from build123d import *

# Parameters (mm, degrees)
SKETCH1_W                 = 50.8
SKETCH1_H                 = 50.8
BOSS_EXTRUDE1_DEPTH       = 79.375
CUT_EXTRUDE1_DEPTH        = 3.175
SKETCH3_R                 = 55.5625
CUT_EXTRUDE2_DEPTH        = 108.059192156
F_8_32_TAPPED_HOLE1_D     = 3.4544
F_8_32_TAPPED_HOLE1_DEPTH = 10.70864
F_8_32_TAPPED_HOLE1_TIP   = 1.037806461
F_8_32_TAPPED_HOLE2_D     = 3.4544
F_8_32_TAPPED_HOLE2_DEPTH = 10.70864
F_8_32_TAPPED_HOLE2_TIP   = 1.037806461


with BuildPart() as part:
    # Sketch1 → Boss-Extrude1 (new body)
    with BuildSketch(Plane(origin=(0, 0, 0), x_dir=(1, 0, 0), z_dir=(0, 1, 0))):
        with Locations((25.4, 25.4)):
            Rectangle(SKETCH1_W, SKETCH1_H)
    extrude(amount=BOSS_EXTRUDE1_DEPTH)

    # Sketch2 → Cut-Extrude1 (cut)
    with BuildSketch(Plane(origin=(0, 79.375, 0), x_dir=(1, 0, 0), z_dir=(0, 1, 0))):
        with BuildLine():
            Line((130.016993909, 125.017737196), (134.25782275, 78.573759143))
            ThreePointArc((134.25782275, 78.573759143), (134.034685181, 75.298190088), (132.798116214, 72.256802214))
            ThreePointArc((132.798116214, 72.256802214), (130.01096738, 66.280890285), (128.580118229, 59.844090402))
            ThreePointArc((128.580118229, 59.844090402), (125.846501332, 47.24207899), (120.576283082, 35.473130329))
            ThreePointArc((120.576283082, 35.473130329), (120.013426501, 34.114565768), (119.824473194, 32.656209898))
            ThreePointArc((119.824473194, 32.656209898), (117.90735564, 28.45485307), (113.469501546, 27.177281171))
            ThreePointArc((113.469501546, 27.177281171), (106.116591491, 23.83727612), (106.198458812, 15.761744078))
            ThreePointArc((106.198458812, 15.761744078), (105.465515747, 8.75311664), (98.443142857, 8.166309094))
            ThreePointArc((98.443142857, 8.166309094), (95.25, 9.168506799), (92.056857143, 8.166309094))
            ThreePointArc((92.056857143, 8.166309094), (88.9, 7.1755), (85.743142857, 8.166309094))
            ThreePointArc((85.743142857, 8.166309094), (82.55, 9.168506799), (79.356857143, 8.166309094))
            ThreePointArc((79.356857143, 8.166309094), (76.212257074, 7.175513597), (73.063291467, 8.152345678))
            ThreePointArc((73.063291467, 8.152345678), (69.907489389, 9.140393728), (66.74574768, 8.171520637))
            ThreePointArc((66.74574768, 8.171520637), (63.508942298, 7.175501389), (60.273525168, 8.176020964))
            ThreePointArc((60.273525168, 8.176020964), (57.10532095, 9.149271709), (53.943097961, 8.156759366))
            ThreePointArc((53.943097961, 8.156759366), (50.791625748, 7.175506347), (47.643142857, 8.166309094))
            ThreePointArc((47.643142857, 8.166309094), (44.45, 9.168506799), (41.256857143, 8.166309094))
            ThreePointArc((41.256857143, 8.166309094), (38.1, 7.1755), (34.943142857, 8.166309094))
            ThreePointArc((34.943142857, 8.166309094), (31.75, 9.168506799), (28.556857143, 8.166309094))
            ThreePointArc((28.556857143, 8.166309094), (25.4, 7.1755), (22.243142857, 8.166309094))
            ThreePointArc((22.243142857, 8.166309094), (19.05, 9.168506799), (15.856857143, 8.166309094))
            ThreePointArc((15.856857143, 8.166309094), (8.793588587, 8.793588587), (8.166309094, 15.856857143))
            ThreePointArc((8.166309094, 15.856857143), (9.168506799, 19.05), (8.166309094, 22.243142857))
            ThreePointArc((8.166309094, 22.243142857), (7.1755, 25.4), (8.166309094, 28.556857143))
            ThreePointArc((8.166309094, 28.556857143), (9.168506799, 31.75), (8.166309094, 34.943142857))
            ThreePointArc((8.166309094, 34.943142857), (7.1755, 38.1), (8.166309094, 41.256857143))
            ThreePointArc((8.166309094, 41.256857143), (9.168506799, 44.45), (8.166309094, 47.643142857))
            ThreePointArc((8.166309094, 47.643142857), (7.175506347, 50.791625748), (8.156759366, 53.943097961))
            ThreePointArc((8.156759366, 53.943097961), (9.149271709, 57.10532095), (8.176020964, 60.273525168))
            ThreePointArc((8.176020964, 60.273525168), (7.175501389, 63.508942298), (8.171520637, 66.74574768))
            ThreePointArc((8.171520637, 66.74574768), (9.140393728, 69.907489389), (8.152345678, 73.063291467))
            ThreePointArc((8.152345678, 73.063291467), (7.175513597, 76.212257074), (8.166309094, 79.356857143))
            ThreePointArc((8.166309094, 79.356857143), (9.168506799, 82.55), (8.166309094, 85.743142857))
            ThreePointArc((8.166309094, 85.743142857), (7.1755, 88.9), (8.166309094, 92.056857143))
            ThreePointArc((8.166309094, 92.056857143), (9.168506799, 95.25), (8.166309094, 98.443142857))
            ThreePointArc((8.166309094, 98.443142857), (8.75311664, 105.465515747), (15.761744078, 106.198458812))
            ThreePointArc((15.761744078, 106.198458812), (23.83727612, 106.116591491), (27.177281171, 113.469501546))
            ThreePointArc((27.177281171, 113.469501546), (28.45485307, 117.90735564), (32.656209898, 119.824473194))
            ThreePointArc((32.656209898, 119.824473194), (34.114565768, 120.013426501), (35.473130329, 120.576283082))
            ThreePointArc((35.473130329, 120.576283082), (47.24207899, 125.846501332), (59.844090402, 128.580118229))
            ThreePointArc((59.844090402, 128.580118229), (68.705211612, 130.952457845), (76.452938417, 135.863689229))
            ThreePointArc((76.452938417, 135.863689229), (80.625736152, 138.0725352), (85.345346996, 138.201045691))
            Line((85.345346996, 138.201045691), (125.626948268, 129.926898817))
            ThreePointArc((125.626948268, 129.926898817), (128.63345164, 128.197989094), (130.016993909, 125.017737196))
        make_face()
    extrude(amount=-CUT_EXTRUDE1_DEPTH, mode=Mode.SUBTRACT)

    # Sketch3 → Cut-Extrude2 (cut, through all)
    with BuildSketch(Plane(origin=(0, 79.375, 0), x_dir=(1, 0, 0), z_dir=(0, 1, 0))):
        with Locations((66.675, 66.675)):
            Circle(SKETCH3_R)
    extrude(amount=-CUT_EXTRUDE2_DEPTH, mode=Mode.SUBTRACT)

    # #8-32 Tapped Hole1
    with Locations(Plane(origin=(393.7, -15.875, 0), x_dir=(1, 0, 0), z_dir=(0, 0, 1))):
        with Locations((-300, 82.55), (-240, 82.55), (-180, 82.55), (-60, 82.55), (0, 82.55), (60, 82.55), (120, 82.55), (180, 82.55), (240, 82.55), (-120, 82.55), (-360, 82.55), (300, 82.55), (360, 82.55)):
            Hole(F_8_32_TAPPED_HOLE1_D / 2, depth=F_8_32_TAPPED_HOLE1_DEPTH)
            with Locations((0, 0, -(F_8_32_TAPPED_HOLE1_DEPTH + F_8_32_TAPPED_HOLE1_TIP / 2))):  # 118° drill point
                Cone(0, F_8_32_TAPPED_HOLE1_D / 2, F_8_32_TAPPED_HOLE1_TIP, mode=Mode.SUBTRACT)

    # #8-32 Tapped Hole2
    with Locations(Plane(origin=(0, -15.875, -393.7), x_dir=(0, 0, 1), z_dir=(-1, 0, 0))):
        with Locations((-300, 82.55), (-240, 82.55), (-180, 82.55), (-60, 82.55), (0, 82.55), (60, 82.55), (120, 82.55), (180, 82.55), (240, 82.55), (-120, 82.55), (-360, 82.55), (300, 82.55), (360, 82.55)):
            Hole(F_8_32_TAPPED_HOLE2_D / 2, depth=F_8_32_TAPPED_HOLE2_DEPTH)
            with Locations((0, 0, -(F_8_32_TAPPED_HOLE2_DEPTH + F_8_32_TAPPED_HOLE2_TIP / 2))):  # 118° drill point
                Cone(0, F_8_32_TAPPED_HOLE2_D / 2, F_8_32_TAPPED_HOLE2_TIP, mode=Mode.SUBTRACT)


solid = part.part
Input: part model. Units: mm. Frame: model coordinates. A direction names the side the tool comes from. Coordinates: 2 decimals unless noted, no trailing zeros. Order: outer loops, then holes, each group sorted by start corner. A loop starts at its lowest first (then second) coordinate and runs counter-clockwise, first axis right, second up. Notation, with made-up numbers: M -39.5,57 L -13.5,57 A17 ccw -13.5,88 Z; hole C 10.5,-22.75 d6. An arc over 180 degrees is marked long. One line per question, with ' | ' between items.
Item 1: Section C-C (x = 27). Output: boundary loops of the cut face in (y, z) (3 decimals), then the cut area to 3 significant figures.
Geometry results:
outline: M 0,-27.777 L 76.2,-27.777 L 76.2,-7.412 L 79.375,-7.412 L 79.375,0 L 0,0 Z | area: 2,140 mm^2
Item 2: Pin query (flat end, axial travel): pin 1 (6 mm diameter, centred on x = 27, y = 56.5, fed in from +Z); pin 2 (2 mm diameter, centred on y = 66.675, z = -33.7, fed in from -X); pin 3 (13 mm diameter, centred on x = 28.5, z = -28.5, fed in from +Y); pin 4 (6 mm diameter, centred on y = 22, z = -38.5, fed in from +X). Return the tip coordinate at first contact, or that it passes through.
Geometry results:
pin 1: stops at z = 0 | pin 2: stops at x = 11.15 | pin 3: stops at y = 76.2 | pin 4: stops at x = 20.68
Item 3: Section A-A (z = -40). Output: boundary loops of the cut face in (x, y) (1 decimal), then the cut area to 3 significant figures.
Geometry results:
outline: M 0,0 L 17.9,0 L 17.9,76.2 L 7.5,76.2 L 7.5,79.4 L 0,79.4 Z | area: 1,390 mm^2
Item 4: Section B-B (y = 21). Output: boundary loops of the cut face in (x, z) (1 decimal).
Geometry results:
outline: M 0,-50.8 L 13.4,-50.8 A55.6 cw 50.8,-13.4 L 50.8,0 L 0,0 Z
Item 5: Draft query along Y for faces 4 (the cylindrical face through (9.17, 77.81, -44.4)), 5 (the cylindrical face through (5.43, 68.39, -33.48)), 6 (the flat face through (24, 76.2, -24)), 7 (the cylindrical face through (32.77, 68.13, -5.43)). Return one class per face: released by +Y, released by -Y, zero draft, split by the parting line, or undercut.
Geometry results:
face 4: zero draft | face 5: undercut | face 6: released by +Y | face 7: undercut
Item 6: Ray query, line 1 along Y through (x, z) = (33.7, -5.25) (3 decimals); line 2 along Y through (x, z) = (19, -32); line 3 along Y through (x, z) = (33, -5) (3 decimals). Return the intervals inside material, ascending.
Geometry results:
line 1: y = 0 to 64.948, 68.402 to 79.375 | line 2: y = 0 to 76.2 | line 3: y = 0 to 65.096, 68.254 to 79.375
Item 7: Reachability of faces 1 (the cylindrical face through (9.17, 77.81, -19)), 2 (the cylindrical face through (38.147, 77.81, -7.176)), 3 (the cylindrical face through (7.436, 77.81, -49.123)) from +Z, -Z, +X, -X, +Y, -Y: full face, straight path, thin tool, end or side. Return the list, or none.
Geometry results:
face 1: +X, +Y | face 2: -Z, +Y | face 3: -Z, +X, +Y
